Could you check a few things on this model? Use its own coordinates, in mm. A direction names the side the tool comes from. Give positions to 0.01 mm unless a question says otherwise; leave off trailing zeros. Loops run counter-clockwise (first coordinate to the right, second up) from the corner with the lowest first, then second, coordinate; pieces in that order, holes last. Notation, with made-up numbers: (56.25, 7) -> (79.25, 7) arc R13 cw to (79.25, 18) -> close; hole circle Ø11 at (13, 32.25). An arc over 180 degrees is marked (long way). Write item = value, one per line. Start each with the question number.
1) I want a section at B-B (z = 24.5). List the corners of the cut face in (x, y) for me, and give its area (3 significant figures).
2) On a 3-axis mill with a long thin cutter (end or side, diameter ignored), from which of +Z, -Z, +X, -X, +Y, -Y can I reach the whole of each face in a straight line? I mean faces 1 (the face through (1.521, -17.527, 32.481)), 2 (the face through (1, 17, 0)), 3 (the face through (1.52, 11.24, 38.7)), 4 (the face through (1.52, 11.24, -38.7)). Say none if no direction works.
3) If we mould it in two halves opening along Y, with no side actions, what happens to faces 5 (the face through (0.71, -17.07, -36.5)), 6 (the face through (1.521, 17.527, -32.481)), 7 (the face through (0, 0, 1)), 8 (the face through (1.48, -20.63, -41.64))? For each: +Y half, -Y half, draft (parallel to the pull), parting line (faces both ways), or undercut.
4) I'm going to push flat-ended pins straight in: pin 1 Ø1.5 at (x, z) = (2, -5.5) entering from +Y; pin 2 Ø1.5 at (x, z) = (0.5, -34.5) entering from -Y; pin 3 Ø0.9 at (x, y) = (2, -4.5) entering from -Z. Where does each tip first touch, or does it pass through?
5) I want a section at C-C (y = -4). List the corners of the cut face in (x, z) for me, and give its area (3 significant figures).
6) I need wall thicknesses on probe 1 along Y at (x, z) = (2.65, 36); probe 2 along Y at (x, z) = (1.2, -37.5); probe 3 along Y at (x, z) = (2.6, -38.5). Which ranges of each line are inside material? Lowest first, please. Write a range as from..to.
7) I want a section at A-A (x = 0.7). List the corners of the cut face in (y, z) for me (3 decimals), and give its area (3 significant figures).
from build123d import *

# Parameters (mm, degrees)
EXTRUDE_1_DEPTH          = 3
FILLET_1_R               = 3
HOLE_WIZARD_1_AT_2_COUNT = 2
HOLE_WIZARD_1_AT_2_PITCH = 34
HOLE_WIZARD_1_AT_3_COUNT = 2
HOLE_WIZARD_1_AT_3_PITCH = 83.623920023
HOLE_WIZARD_1_AT_4_COUNT = 2
HOLE_WIZARD_1_AT_4_PITCH = 76.4


with BuildPart() as part:
    # 草图1 → 凸台-拉伸1 (new body)
    with BuildSketch(Plane(origin=(0, 0, 0), x_dir=(0, 0, -1), z_dir=(1, 0, 0))):
        with BuildLine():
            Line((-38.2, 12), (-38.2, -12))
            ThreePointArc((-38.2, -12), (-41.735533906, -20.535533906), (-33.2, -17))
            Line((-33.2, -17), (33.2, -17))
            ThreePointArc((33.2, -17), (41.735533906, -20.535533906), (38.2, -12))
            Line((38.2, -12), (38.2, 12))
            ThreePointArc((38.2, 12), (41.735533906, 20.535533906), (33.2, 17))
            Line((33.2, 17), (-33.2, 17))
            ThreePointArc((-33.2, 17), (-41.735533906, 20.535533906), (-38.2, 12))
        make_face()
    extrude(amount=EXTRUDE_1_DEPTH)

    # 圆角1
    fillet_1_edges = [part.edges().sort_by_distance(p)[0] for p in [
        (1.5, 17, 33.2),
        (1.5, 17, -33.2),
        (1.5, 12, -38.2),
        (1.5, -12, -38.2),
        (1.5, -17, -33.2),
        (1.5, -17, 33.2),
        (1.5, -12, 38.2),
        (1.5, 12, 38.2),
    ]]
    fillet(fillet_1_edges, radius=FILLET_1_R)

    # 草图2 → 打孔尺寸(%根据十字)槽半沉头木螺钉的类型1 (revolve, cut)
    with BuildSketch(Plane(origin=(3, 17, 38.2), x_dir=(0, 0, -1), z_dir=(0, 1, 0))):
        Polygon((0, 0), (0, 3), (1.7, 3), (1.7, 1.6), (3.3, 0), align=None)
    hole_wizard_1 = revolve(axis=Axis((9.35, 17, 38.2), (-1, 0, 0)), mode=Mode.SUBTRACT)

    # 打孔尺寸(%根据十字)槽半沉头木螺钉的类型1 at 2: 打孔尺寸(%根据十字)槽半沉头木螺钉的类型1 ×2
    with Locations(*[(0, -i * HOLE_WIZARD_1_AT_2_PITCH, 0) for i in range(1, HOLE_WIZARD_1_AT_2_COUNT)]):
        add(hole_wizard_1, mode=Mode.SUBTRACT)

    # 打孔尺寸(%根据十字)槽半沉头木螺钉的类型1 at 3: 打孔尺寸(%根据十字)槽半沉头木螺钉的类型1 ×2
    with Locations(*[Vector(0, -0.406582231, -0.913614191) * (i * HOLE_WIZARD_1_AT_3_PITCH) for i in range(1, HOLE_WIZARD_1_AT_3_COUNT)]):
        add(hole_wizard_1, mode=Mode.SUBTRACT)

    # 打孔尺寸(%根据十字)槽半沉头木螺钉的类型1 at 4: 打孔尺寸(%根据十字)槽半沉头木螺钉的类型1 ×2
    with Locations(*[(0, 0, -i * HOLE_WIZARD_1_AT_4_PITCH) for i in range(1, HOLE_WIZARD_1_AT_4_COUNT)]):
        add(hole_wizard_1, mode=Mode.SUBTRACT)


solid = part.part
Answer list:
q1.outline = (0, -17) -> (3, -17) -> (3, 17) -> (0, 17) -> close
q1.area = 102 mm^2
q2.face_1 = +X, -X, -Y
q2.face_2 = +X, -X, +Y
q2.face_3 = +Z, +X, -X
q2.face_4 = -Z, +X, -X
q3.face_5 = undercut
q3.face_6 = +Y half
q3.face_7 = draft
q3.face_8 = undercut
q4.pin_1 = 17
q4.pin_2 = -21.04
q4.pin_3 = -38.2
q5.outline = (0, -38.2) -> (3, -38.2) -> (3, 38.2) -> (0, 38.2) -> close
q5.area = 229 mm^2
q6.probe_1 = -21.49..-18.97, -15.03..15.03, 18.97..21.49
q6.probe_2 = -21.95..-18.55, -15.45..15.45, 18.55..21.95
q6.probe_3 = -21.99..-19.88, -14.12..-10.89, 10.89..14.12, 19.88..21.99
q7.outline = (-18.875, -33.565) arc R5 ccw (long way) to (-12.365, -40.075) arc R3 cw to (-9.584, -38.2) -> (9.584, -38.2) arc R3 cw to (12.365, -40.075) arc R5 ccw (long way) to (18.875, -33.565) arc R3 cw to (17, -30.784) -> (17, 30.784) arc R3 cw to (18.875, 33.565) arc R5 ccw (long way) to (12.365, 40.075) arc R3 cw to (9.584, 38.2) -> (-9.584, 38.2) arc R3 cw to (-12.365, 40.075) arc R5 ccw (long way) to (-18.875, 33.565) arc R3 cw to (-17, 30.784) -> (-17, -30.784) arc R3 cw to start; hole circle Ø3.4 at (-17, -38.2); hole circle Ø3.4 at (-17, 38.2); hole circle Ø3.4 at (17, -38.2); hole circle Ø3.4 at (17, 38.2)
q7.area = 2,800 mm^2
